```python
from build123d import *

# Parameters (mm, degrees)
F0_W      = 34.29
F0_H      = 34.29
F1_DEPTH  = 34.29
F2_R      = 12.7
F3_DEPTH  = 50.8
F4_R      = 3.429
F5_DEPTH  = 25.4
F6_R      = 3.429
F7_DEPTH  = 25.4
F8_R      = 3.429
F9_DEPTH  = 25.4
F10_R     = 2.54
F11_R     = 12.7
F12_DEPTH = 50.8
F13_R     = 3.429
F14_DEPTH = 25.4
F15_R     = 3.429
F16_DEPTH = 25.4
F17_R     = 12.7
F18_DEPTH = 50.8
F19_R     = 2.032
F20_R     = 3.429
F21_DEPTH = 25.4


with BuildPart() as f1:
    # F0 (on Top) → F1 (new body)
    with BuildSketch(Plane.XY):
        with Locations((3.6728888822, 6.5610635031)):
            Rectangle(F0_W, F0_H)
    extrude(amount=F1_DEPTH)

    # F2 (on face) → F3 (join)
    with BuildSketch(Plane.XZ.offset(10.5839364969)):
        with Locations((3.6728888822, 17.145)):
            Circle(F2_R)
    extrude(amount=F3_DEPTH)

    # F4 (on Front) → F5 (cut, symmetric)
    with BuildSketch(Plane.XZ):
        with Locations((3.6728888822, 53.34)):
            Circle(F4_R)
        with Locations((3.6728888822, 72.39)):
            Circle(F4_R)
    extrude(amount=F5_DEPTH, both=True, mode=Mode.SUBTRACT)

    # F6 (on Right) → F7 (cut, symmetric)
    with BuildSketch(Plane.YZ):
        with Locations((-29.6339364969, 17.145)):
            Circle(F6_R)
        with Locations((-48.6839364969, 17.145)):
            Circle(F6_R)
    extrude(amount=F7_DEPTH, both=True, mode=Mode.SUBTRACT)

    # F8 (on Front) → F9 (cut, symmetric)
    with BuildSketch(Plane.XZ):
        with Locations((-51.5721111178, 17.145)):
            Circle(F8_R)
        with Locations((-32.5221111178, 17.145)):
            Circle(F8_R)
    extrude(amount=F9_DEPTH, both=True, mode=Mode.SUBTRACT)

    # F10
    f10_edges = [f1.edges().sort_by_distance(p)[0] for p in [
        (20.817889, 23.706064, 17.145),
        (20.817889, 6.561064, 34.29),
        (20.817889, -10.583936, 17.145),
        (20.817889, 6.561064, 0),
        (3.672889, 23.706064, 0),
        (3.672889, 23.706064, 34.29),
        (-13.472111, 23.706064, 17.145),
        (-13.472111, 6.561064, 0),
        (3.672889, -10.583936, 0),
        (-13.472111, 6.561064, 34.29),
        (-13.472111, -10.583936, 17.145),
        (3.672889, -10.583936, 34.29),
    ]]
    fillet(f10_edges, radius=F10_R)

    # F11 (on face) → F12 (join)
    with BuildSketch(Plane(origin=(0, 23.7060635031, 0), x_dir=(-1, 0, 0), z_dir=(0, 1, 0))):
        with Locations((-3.6728888822, 17.145)):
            Circle(F11_R)
    extrude(amount=F12_DEPTH)

    # F13 (on Right) → F14 (cut, symmetric)
    with BuildSketch(Plane.YZ):
        with Locations((42.7560635031, 17.145)):
            Circle(F13_R)
        with Locations((61.8060635031, 17.145)):
            Circle(F13_R)
    extrude(amount=F14_DEPTH, both=True, mode=Mode.SUBTRACT)

    # F15 (on Front) → F16 (cut, symmetric)
    with BuildSketch(Plane.XZ):
        with Locations((58.9178888822, 17.145)):
            Circle(F15_R)
        with Locations((39.8678888822, 17.145)):
            Circle(F15_R)
    extrude(amount=F16_DEPTH, both=True, mode=Mode.SUBTRACT)

    # F17 (on face) → F18 (join)
    with BuildSketch(Plane(origin=(0, 0, 0), x_dir=(1, 0, 0), z_dir=(0, 0, -1))):
        with Locations((3.6728888822, -6.5610635031)):
            Circle(F17_R)
    extrude(amount=F18_DEPTH)

    # F19
    f19_edges = [f1.edges().sort_by_distance(p)[0] for p in [
        (-9.027111, -61.383936, 17.145),
        (16.372889, 74.506064, 17.145),
        (-9.027111, 6.561064, -50.8),
    ]]
    fillet(f19_edges, radius=F19_R)

    # F20 (on Right) → F21 (cut, symmetric)
    with BuildSketch(Plane.YZ):
        with Locations((7.0114927366, -19.05)):
            Circle(F20_R)
        with Locations((7.0114927366, -38.1)):
            Circle(F20_R)
    extrude(amount=F21_DEPTH, both=True, mode=Mode.SUBTRACT)


solid = f1.part
```
Part model, mm, in its own coordinate system. A direction names the side the tool comes from. Give positions to 0.01 mm unless a question says otherwise; leave off trailing zeros. Order: outer loops, then holes, each group sorted by start corner. A loop starts at its lowest first (then second) coordinate and runs counter-clockwise, first axis right, second up. Notation, with made-up numbers: (-10.75, 14) - (21.25, 14) arc R16 ccw to (21.25, 36) - close; hole circle Ø7 at (-14.75, 63). An arc over 180 degrees is marked (long way). Use one line per item in the form item = value.
Item 1: Slice it at A-A on y = 5. Count the separate pieces of the cut face and the enclosed holes in it, and give its area (3 significant figures).
Solution:
separate_pieces = 3
enclosed_holes = 0
area = 2,170 mm2
Item 2: Probe probe 1 along Y at (x, z) = (7.5, 20); probe 2 along Y at (x, z) = (17, 20); probe 3 along Y at (x, z) = (0, -38). List the from-to ranges inside material, lowest first. Write a range as from..to.
Solution:
probe_1 = -61.38..-50.58, -46.78..-31.53, -27.73..40.86, 44.66..59.91, 63.71..74.51
probe_2 = -10.58..23.71
probe_3 = -5.6..3.58, 10.44..18.72
Item 3: Which spindle directions (+Z, -Z, +X, -X, +Y, -Y) get a long thin tool onto all of the face, cutting with end or side? Do faces 5 (the face through (-8.06, 47.75, 12.28)), 6 (the face through (15.404, 11.425, -24.043)), 7 (the face through (3, -10.584, 30)). Say none if no direction does.
Solution:
face_5 = +Y
face_6 = -Z
face_7 = -Y
Item 4: Slice it at B-B on z = -40. Give the cut face in (x, y), and give its area (3 significant figures).
Solution:
outline = (-8.8, 4.16) arc R12.7 ccw to (16.14, 4.16) - close; (-8.59, 9.87) - (15.94, 9.87) arc R12.7 ccw to start
area = 363 mm2
Item 5: Pin check, flat tips, straight feed: pin 1 Ø12 at (x, y) = (8.5, -42.5) entering from -Z (3 decimals); pin 2 Ø1 at (x, z) = (10, -20) entering from +Y; pin 3 Ø10 at (y, z) = (4, -39) entering from -X; pin 4 Ø6 at (y, z) = (7.01, -19.05) entering from -X. Stop position of each tip, or through.
Solution:
pin_1 = 4.445
pin_2 = 17.85
pin_3 = -9.03
pin_4 = through
Item 6: Two-plate mould, pull along Z, no slides. Class faces 1 (the face through (-12.748, 6.766, 0.764)), 2 (the face through (20.818, 6, 17)), 3 (the face through (20.05, 6.77, 33.57)), 4 (the face through (3.847, -51.211, 19.462)): released by +Z, released by -Z, zero draft, split by the parting line, or undercut.
Solution:
face_1 = released by -Z
face_2 = zero draft
face_3 = released by +Z
face_4 = undercut
